```python
from build123d import *

# Parameters (mm, degrees)
F0_R     = 1.5
F0_R_2   = 14.25
F1_DEPTH = 6
F2_R     = 1.5
F3_DEPTH = 30.251
F4_R     = 2.5


with BuildPart() as f1:
    # F0 (on Top) → F1 (new body)
    with BuildSketch(Plane.XY):
        with BuildLine():
            ThreePointArc((-10, 17.608592), (-10.187308, -17.500893), (20.25, 0))
            ThreePointArc((20.25, 0), (17.500893, 10.187308), (10, 17.608592))
            ThreePointArc((10, 17.608592), (8.52849, 18.366474), (7, 19.001645))
            ThreePointArc((7, 19.001645), (0, 20.25), (-7, 19.001645))
            ThreePointArc((-7, 19.001645), (-8.52849, 18.366474), (-10, 17.608592))
        make_face()
        with Locations((-13.214267, -11.088086)):
            Circle(F0_R, mode=Mode.SUBTRACT)
        with Locations((13.214267, -11.088086)):
            Circle(F0_R, mode=Mode.SUBTRACT)
        Circle(F0_R_2, mode=Mode.SUBTRACT)
        with BuildLine():
            ThreePointArc((-11.714267, 11.088086), (-11.804728, 10.575056), (-12.0652, 10.123905))
            ThreePointArc((-12.0652, 10.123905), (-14.178448, 9.93902), (-14.363333, 12.052268))
            ThreePointArc((-14.363333, 12.052268), (-12.701236, 12.497625), (-11.714267, 11.088086))
        make_face(mode=Mode.SUBTRACT)
        with BuildLine():
            ThreePointArc((14.714267, 11.088086), (13.727297, 9.678547), (12.0652, 10.123905))
            ThreePointArc((12.0652, 10.123905), (12.250085, 12.237153), (14.363333, 12.052268))
            ThreePointArc((14.363333, 12.052268), (14.623806, 11.601116), (14.714267, 11.088086))
        make_face(mode=Mode.SUBTRACT)
        with BuildLine():
            ThreePointArc((7, 19.001645), (8.52849, 18.366474), (10, 17.608592))
            Line((10, 17.608592), (10, 27.25))
            Line((10, 27.25), (7, 27.25))
            Line((7, 27.25), (7, 19.001645))
        make_face()
        with BuildLine():
            Line((-10, 27.25), (-10, 17.608592))
            ThreePointArc((-10, 17.608592), (-8.52849, 18.366474), (-7, 19.001645))
            Line((-7, 19.001645), (-7, 27.25))
            Line((-7, 27.25), (-10, 27.25))
        make_face()
    extrude(amount=F1_DEPTH)

    # F2 (on face) → F3 (cut, through all)
    with BuildSketch(Plane(origin=(-10, 0, 0), x_dir=(0, -1, 0), z_dir=(-1, 0, 0))):
        with Locations((-23.861416, 3)):
            Circle(F2_R)
    extrude(amount=-F3_DEPTH, mode=Mode.SUBTRACT)

    # F4
    f4_edges = [f1.edges().sort_by_distance(p)[0] for p in [
        (8.5, 27.25, 6),
        (8.5, 27.25, 0),
        (-8.5, 27.25, 0),
        (-8.5, 27.25, 6),
    ]]
    fillet(f4_edges, radius=F4_R)


solid = f1.part
```
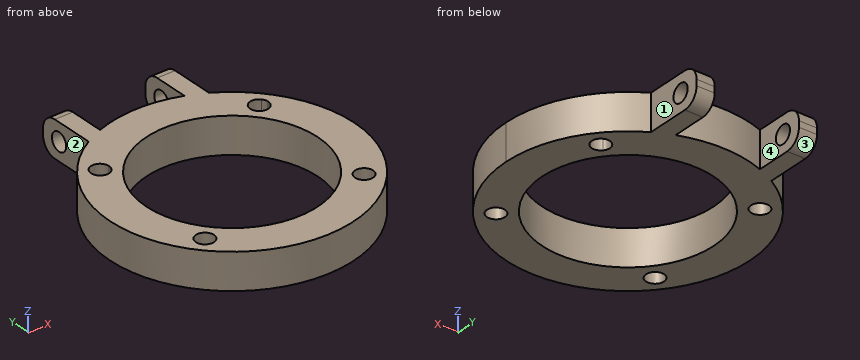
Check sheet for the modelled part. Datum: model origin and axes. Units: mm. Face numbers are marked on the shaded views. Coordinates: 2 decimals unless noted, no trailing zeros. Order: outer loops, then holes, each group sorted by start corner. A loop starts at its lowest first (then second) coordinate and runs counter-clockwise, first axis right, second up. Notation, with made-up numbers: (-16.5, -34) -> (-8.5, -34) arc R16 cw to (-8.5, -21) -> close; hole circle Ø6 at (69.25, 0). An arc over 180 degrees is marked (long way). Write each question's results on one line, items separated by ' | '. Start each with the question number.
1) Draft check along X on the marked faces 1, 2, 3 and 4. Enter one of: pulls with the +X half, pulls with the -X half, needs draft (parallel to the pull), parting line crosses it, or undercut.
2) Section check D-D (z = 0.7). Enter the section's corners in (x, y), and give its area (3 significant figures).
3) Section check B-B (y = -8). Enter the section's corners in (x, z), and give its area (3 significant figures).
4) Section check C-C (y = 23). Enter the section's corners in (x, z).
5) Depth check by flat-ended pin: pin 1 (3.5 mm diameter, centred on x = 13.21, y = -11.09, fed in from +Z); pin 2 (1.8 mm diameter, centred on y = 22.5, z = 3.5, fed in from -X); pin 3 (3 mm diameter, centred on x = 7, z = 5, fed in from -Y); pin 4 (10 mm diameter, centred on x = -1, y = -8, fed in from +Z). Enter the tip coordinate at first touch or a pass-through.
6) Section check A-A (x = 11). Enter the section's corners in (y, z), and give its area (3 significant figures).
7) Material ranges on line 1 along Y through (x, z) = (-12.5, 5.2); line 2 along X through (y, z) = (21.5, 5.6); line 3 along Y through (x, z) = (4, 0.4), recorded low to high.
Checked values:
1) face 1: pulls with the +X half | face 2: pulls with the -X half | face 3: needs draft | face 4: undercut
2) outline: (-10, 17.61) arc R20.25 ccw (long way) to (10, 17.61) -> (10, 26.48) -> (7, 26.48) -> (7, 19) arc R20.25 ccw to (-7, 19) -> (-7, 26.48) -> (-10, 26.48) -> close; hole circle Ø3 at (-13.21, -11.09); hole circle Ø3 at (-13.21, 11.09); hole circle Ø28.5 at (0, 0); hole circle Ø3 at (13.21, -11.09); hole circle Ø3 at (13.21, 11.09) | area: 671 mm²
3) outline: (-18.6, 0) -> (-11.79, 0) -> (-11.79, 6) -> (-18.6, 6) -> close; (11.79, 0) -> (18.6, 0) -> (18.6, 6) -> (11.79, 6) -> close | area: 81.7 mm²
4) outline: (-10, 0) -> (-7, 0) -> (-7, 1.77) -> (-10, 1.77) -> close; (-10, 4.23) -> (-7, 4.23) -> (-7, 6) -> (-10, 6) -> close; (7, 0) -> (10, 0) -> (10, 1.77) -> (7, 1.77) -> close; (7, 4.23) -> (10, 4.23) -> (10, 6) -> (7, 6) -> close
5) pin 1: z = 6 | pin 2: x = -10 | pin 3: y = -19.49 | pin 4: through
6) outline: (-17, 0) -> (-9.06, 0) -> (-9.06, 6) -> (-17, 6) -> close; (9.06, 0) -> (17, 0) -> (17, 6) -> (9.06, 6) -> close | area: 95.3 mm²
7) line 1: -15.93 to -12.41, -9.77 to -6.84, 6.84 to 9.77, 12.41 to 15.93 | line 2: -10 to -7, 7 to 10 | line 3: -19.85 to -13.68, 13.68 to 19.85
